Autodesk Inventor part; units mm, degrees
ref_plane "Work Plane1" through (-25, 0, 0) normal (1, 0, 0) x (0, 1, 0)
ref_plane "Work Plane2" through (0, 2.5, 0) normal (0, 1, 0) x (-1, 0, 0)
ref_plane "XY Plane" through (0, 0, 0) normal (0, 0, 1) x (1, 0, 0)
sketch "Sketch1" plane through (0, 0, 0) normal (0, 1, 0) x (-1, 0, 0)
  arc A0 (25, 0) -> (-24.98, 1) centre (0, 0) ccw
  arc A1 (24, 0) -> (-24, 0) centre (0, 0) ccw
  line L0 (25, 0) -> (24, 0)
  line L1 (-24, 0) -> (-25, 0)
  line L2 (-24, 0) -> (-29.5, 0)
  line L3 (-29.5, 0) -> (-29.5, 1)
  line L4 (-29.5, 1) -> (-24.98, 1)
  line L5 (-24, 1) -> (-24, 0)
extrude "Extrusion1" add sketch "Sketch1" along normal blind 5
sketch "Sketch2" plane through (29.5, 0, 0) normal (0, 0, -1) x (-1, 0, 0)
  line L0 (0, 0) -> (5.5, 0)
  arc A0 (2.5, 5) -> (2.5, 0) centre (2.5, 2.5) ccw
  line L1 (0, 0) -> (2.5, 0)
  line L2 (4.52, 0) -> (0, 0)
  line L3 (0, 0) -> (0, 2.5)
  line L4 (0, 0) -> (0, 5)
  line L5 (0, 2.5) -> (0, 5)
  line L6 (0, 5) -> (2.26, 5)
  line L7 (4.52, 5) -> (0, 5)
  line L8 (2.5, 5) -> (0, 5)
  line L9 (0, 2.5) -> (0, 5)
  line L10 (0, 2.5) -> (0, 0)
  line L11 (0, 0) -> (2.5, 0)
  arc A1 (0, 2.5) -> (2.5, 0) centre (2.5, 2.5) ccw
  arc A2 (2.5, 5) -> (0, 2.5) centre (2.5, 2.5) ccw
  point P0 (29.5, 0)
extrude "Extrusion2" cut sketch "Sketch2" against normal through all
ref_plane "Work Plane1" through (-25, 0, 0) normal (1, 0, 0) x (0, 1, 0)
sketch "Sketch3" plane through (-25, 0, 0) normal (1, 0, 0) x (0, 1, 0)
  line L0 (5, 0) -> (5, 25) construction
  line L1 (0, 0) -> (0, 2) construction
  line L2 (0, 0) -> (0, 25) construction
  line L3 (0, 0) -> (0, 2.5) construction
  arc A0 (0, 2.5) -> (5, 2.5) centre (2.5, 2.5) ccw
  line L4 (0, 0) -> (0, 2.5)
  line L5 (0, 0) -> (5, 0)
  line L6 (0, 0) -> (2.5, 0)
  line L7 (2.5, 0) -> (5, 0)
  line L8 (5, 0) -> (5, 2.5)
  arc A1 (0, 2.5) -> (2.5, 0) centre (2.5, 2.5) ccw
  arc A2 (2.5, 0) -> (5, 2.5) centre (2.5, 2.5) ccw
  point P0 (0, 1)
  point P1 (5, 1)
extrude "Extrusion3" cut sketch "Sketch3" along normal blind 3
sketch "Sketch4" plane through (-25, 0, 0) normal (1, 0, 0) x (0, 1, 0)
  line L0 (0, 0) -> (0, 4.5) construction
  line L1 (0, 24) -> (0, 0) construction
  line L2 (0, 4.5) -> (5, 4.5) construction
  line L3 (5, 24) -> (5, 0) construction
  circle A0 centre (2.5, 4.5) radius 1.5
  point P0 (0, 2.5)
  point P1 (5, 2.5)
  dimension "d15" = 4.5
  dimension "d16" = 3
extrude "Extrusion4" cut sketch "Sketch4" along normal blind 4
ref_plane "Work Plane2" through (0, 2.5, 0) normal (0, 1, 0) x (-1, 0, 0)
sketch "Sketch6" plane through (0, 2.5, 0) normal (0, 1, 0) x (-1, 0, 0)
  arc A0 (25.04, 7) -> (-25.04, 7) centre (0, 0) ccw
  line L0 (23.9792, 7) -> (25.04, 7)
  line L1 (-23.9792, 7) -> (-25.04, 7)
  arc A1 (23.9792, 7) -> (-23.9792, 7) centre (0, 0) ccw
  point P0 (0, 7)
  dimension "d22" = 52
  dimension "d23" = 7
extrude "Extrusion5" add sketch "Sketch6" along normal mid plane 3
properties part number "Metal icecream cutter"
Can you work these out from the model? Positions are in its coordinate system, mm. A direction names the side the tool comes from. Round coordinates to 2 decimals unless told otherwise and drop trailing zeros. Write each loop counter-clockwise with the first axis right and the second up, starting at its lowest first coordinate (ties: lowest second). Pieces come first, ordered by that corner, then holes. Notation, with made-up numbers: M 68,43.25 L 109,43.25 A32 cw 109,72.25 Z; hole C 0.25,30.25 d1. An arc over 180 degrees is marked long. Use CSV: the item, a comma, the result in double quotes.
(1) Imagine slicing it at B-B (y = 1.5). Write out the boundary of the cut face in (x, z), plus the area to 3 significant figures.
Check values:
outline,"M -25.04,7 L -24,7 A25 ccw -24.36,5.62 L -23.33,5.62 A24 cw 24,0 L 29.29,0 L 29.29,1 L 24.98,1 A25 ccw 24,7 L 25.04,7 A26 ccw Z; M -25,0.21 L -24,0.21 A24 cw -23.76,3.38 L -24.77,3.38 A25 ccw Z"
area,"145 mm^2"
(2) I need wall thicknesses on line 1 along Y through (x, z) = (-24, 4.5); line 2 along X through (y, z) = (0.65, 16); line 3 along X through (y, z) = (2.45, 11.25). Which ranges of each line are inside material? Lowest first, please.
Check values:
line 1,"0 to 1, 4 to 5"
line 2,"-19.21 to -17.89, 17.89 to 19.21"
line 3,"-23.44 to -21.2, 21.2 to 23.44"
(3) Imagine slicing it at C-C (z = 20). Write out the boundary of the cut face in (x, y).
Check values:
outline,"M -16.61,1 L -15,1 L -15,0 L -13.27,0 L -13.27,5 L -15,5 L -15,4 L -16.61,4 Z; M 13.27,0 L 15,0 L 15,1 L 16.61,1 L 16.61,4 L 15,4 L 15,5 L 13.27,5 Z"
(4) I'm going to push flat-ended pins straight in: pin 1 (1.4 mm diameter, centred on x = 27.5, y = 2, fed in from +Z); pin 2 (0.8 mm diameter, centred on x = 24.5, y = 3, fed in from -Z); pin 3 (6 mm diameter, centred on x = -17.5, z = 10, fed in from -Y); pin 4 (2 mm diameter, centred on x = 8.5, y = 1, fed in from -Z). Where does each tip first touch, or does it pass through?
Check values:
pin 1,"z = 1"
pin 2,"z = 0"
pin 3,"through"
pin 4,"z = 22.04"
(5) On a 3-axis mill with a long thin cutter (end or side, diameter ignored), from which of +Z, -Z, +X, -X, +Y, -Y can I reach the whole of each face in a straight line? I mean faces 5 (the cylindrical face through (-24.04, 2.305, 3.013)), 6 (the cylindrical face through (-24.4, 2.6, 0)), 7 (the flat face through (0.1, 1, 25.7)), 8 (the flat face through (0.1, 4, 25.7)). Say none if no direction works.
Check values:
face 5,"-X"
face 6,"-Z, -X"
face 7,"+Z, -Y"
face 8,"+Z, +Y"
(6) We'd pull the mould along X, two halves only. Please class faces 1 (the cylindrical face through (29.5, 2.6, 0.5)), 2 (the cylindrical face through (0.527, 2.465, 23.994)), 3 (the flat face through (5, 5, 24)), 4 (the cylindrical face through (0, 2, 26)): +X half, -X half, draft (parallel to the pull), parting line (faces both ways), or undercut.
Check values:
face 1,"+X half"
face 2,"undercut"
face 3,"draft"
face 4,"parting line"
(7) Imagine slicing it at D-D (x = -2). Write out the boundary of the cut face in (y, z).
Check values:
outline,"M 0,23.92 L 5,23.92 L 5,24.92 L 4,24.92 L 4,25.92 L 1,25.92 L 1,24.92 L 0,24.92 Z"
(8) Imagine slicing it at A-A (z = 4.5). Write out the boundary of the cut face in (x, y).
Check values:
outline,"M -24.59,0 L -23.57,0 L -23.57,1 L -24.59,1 Z; M -24.59,4 L -23.57,4 L -23.57,5 L -24.59,5 Z; M 23.57,0 L 24.59,0 L 24.59,5 L 23.57,5 Z"
